```python
from build123d import *

# Parameters (mm, degrees)
ESBO_O1_W                        = 45
ESBO_O1_H                        = 45
RESSALTO_EXTRUS_O1_DEPTH         = 20
ESBO_O2_W                        = 25
ESBO_O2_H                        = 25
CORTE_EXTRUS_O1_DEPTH            = 70.705238631
ESBO_O3_W                        = 20
ESBO_O3_H                        = 20
RESSALTO_EXTRUS_O2_DEPTH         = 25
FURO_DE_DI_METRO_6_2_6_2_1_D     = 6.2
FURO_DE_DI_METRO_6_2_6_2_1_DEPTH = 35
FURO_DE_DI_METRO_6_2_6_2_2_D     = 6.2
FURO_DE_DI_METRO_6_2_6_2_2_DEPTH = 35
FURO_DE_DI_METRO_6_2_6_2_3_D     = 6.2
FURO_DE_DI_METRO_6_2_6_2_3_DEPTH = 35
FILETE2_R                        = 8
CHANFRO1_SIZE                    = 25
CHANFRO2_SIZE                    = 25
RESSALTO_EXTRUS_O3_DEPTH         = 20
ESBO_O12_R                       = 3
CORTE_EXTRUS_O2_DEPTH            = 71.906960985


# Some blends are built 0.0001 mm under size
with BuildPart() as part:
    # Esboço1 → Ressalto-extrusão1 (new body)
    with BuildSketch(Plane.XY.offset(20)):
        with Locations((-12.862035225, 34.142270059)):
            Rectangle(ESBO_O1_W, ESBO_O1_H)
    extrude(amount=-RESSALTO_EXTRUS_O1_DEPTH)

    # Esboço2 → Corte-extrusão1 (cut, through all)
    with BuildSketch(Plane(origin=(0, 0, 0), x_dir=(-1, 0, 0), z_dir=(0, 0, -1))):
        with Locations((2.862035225, 44.142270059)):
            Rectangle(ESBO_O2_W, ESBO_O2_H)
    extrude(amount=-CORTE_EXTRUS_O1_DEPTH, mode=Mode.SUBTRACT)

    # Esboço3 → Ressalto-extrusão2 (add)
    with BuildSketch(Plane.XY.offset(20)):
        with Locations((-25.362035225, 21.642270059)):
            Rectangle(ESBO_O3_W, ESBO_O3_H)
    extrude(amount=RESSALTO_EXTRUS_O2_DEPTH)

    # Furo de diâmetro Ø6.2 (6.2)1
    with Locations(Plane(origin=(9.637964775, 0, 0), x_dir=(0, 0, -1), z_dir=(1, 0, 0))):
        with Locations((-10, 21.642270059)):
            Hole(FURO_DE_DI_METRO_6_2_6_2_1_D / 2, depth=FURO_DE_DI_METRO_6_2_6_2_1_DEPTH)

    # Furo de diâmetro Ø6.2 (6.2)2
    with Locations(Plane(origin=(0, 56.642270059, 0), x_dir=(1, 0, 0), z_dir=(0, 1, 0))):
        with Locations((-25.362035225, -10)):
            Hole(FURO_DE_DI_METRO_6_2_6_2_2_D / 2, depth=FURO_DE_DI_METRO_6_2_6_2_2_DEPTH)

    # Furo de diâmetro Ø6.2 (6.2)3
    with Locations(Plane.XY.offset(45)):
        with Locations((-25.362035225, 21.642270059)):
            Hole(FURO_DE_DI_METRO_6_2_6_2_3_D / 2, depth=FURO_DE_DI_METRO_6_2_6_2_3_DEPTH)

    # Filete2
    filete2_edges = [part.edges().sort_by_distance(p)[0] for p in [
        (-35.362035225, 34.142270059, 0),
        (-12.862035225, 11.642270059, 0),
        (-35.362035225, 11.642270059, 22.5),
    ]]
    fillet(filete2_edges, radius=FILETE2_R)

    # Chanfro1
    # the kernel refuses this chamfer: 25 mm, written as the material it adds along each edge
    with BuildSketch(Plane(origin=(-35.362035225, 31.642270059, 20), x_dir=(0, -0.027495876610586317, 0.9996219169112966), z_dir=(1, 0, 0))) as chanfro1_piece_1_section:
        Polygon((CHANFRO1_SIZE * 0.999621916911, -CHANFRO1_SIZE * 0.0274958766106), (-CHANFRO1_SIZE * 0.0274958766106, -CHANFRO1_SIZE * 0.999621916911), (0, 0), align=None)
    chanfro1_piece_1 = extrude(amount=20, mode=Mode.PRIVATE)
    chanfro1_piece_1 = split(chanfro1_piece_1, bisect_by=Plane(origin=(-25.362035225, 39.873368248, 45), z_dir=(0, 0, -1)), keep=Keep.TOP, mode=Mode.PRIVATE)
    chanfro1_piece_1 = split(chanfro1_piece_1, bisect_by=Plane(origin=(-25.362035225, 56.642270059, 28.231098189), z_dir=(0, -1, 0)), keep=Keep.TOP, mode=Mode.PRIVATE)
    add(chanfro1_piece_1)

    # Chanfro2
    chanfro2_edges = [part.edges().sort_by_distance(p)[0] for p in [
        (-15.362035225, 31.642270059, 10),
    ]]
    chamfer(chanfro2_edges, length=CHANFRO2_SIZE - 0.0001)  # a hair under: the kernel refuses the full size

    # Esboço10 → Ressalto-extrusão3 (add)
    with BuildSketch(Plane.XZ.offset(-11.642270059)):
        Polygon((-15.362035225, 45), (9.637964775, 20), (-15.362035225, 20), align=None)
    extrude(amount=-RESSALTO_EXTRUS_O3_DEPTH)

    # Esboço12 → Corte-extrusão2 (cut, through all)
    with BuildSketch(Plane(origin=(20.426744945, 20.426744945, 20.426744945), x_dir=(-0.8164965809277259, 0.408248290463863, 0.4082482904638632), z_dir=(-0.577350269189626, -0.5773502691896256, -0.5773502691896258))):
        with Locations(Location((33.625917704, 8.232328107, 0), (0, 0, 120.000005232))):
            Circle(ESBO_O12_R)
    extrude(amount=CORTE_EXTRUS_O2_DEPTH, mode=Mode.SUBTRACT)


solid = part.part
```
Check sheet for the modelled part. Datum: model origin and axes. Units: mm. A direction names the side the tool comes from. Round coordinates to 2 decimals unless told otherwise and drop trailing zeros. Order: outer loops, then holes, each group sorted by start corner. A loop starts at its lowest first (then second) coordinate and runs counter-clockwise, first axis right, second up. Notation, with made-up numbers: M 12.5,34 L 52.5,34 A8 ccw 52.5,48 Z; hole C 58.25,-27.75 d9. An arc over 180 degrees is marked long. Answer in a Markdown table with one row per item.
(1) Section check B-B on y = 52.5. Record the boundary of the cut face in (x, z), plus the area to 3 significant figures.
Findings:
| item | result |
|---|---|
| outline | M -35.36,8 A8 ccw -27.36,0 L -11.22,0 L -11.22,20 L -15.36,20 L -15.36,24.14 L -35.36,24.14 Z; hole C -25.36,10 d6.2 |
| area | 522 mm^2 |
(2) Set-up check for faces 5 (the cylindrical face through (-28.226, 20.455, 27.58)), 6 (the cylindrical face through (-26.81, 15.99, 6.93)), 7 (the cylindrical face through (-7.782, 19.756, 7.54)), 8 (the flat face through (-8, 31.642, 27)), 9 (the cylindrical face through (-27.029, 39.222, 7.386)): record each of +Z, -Z, +X, -X, +Y, -Y from which the full face is reachable in a straight line by a thin tool's end or side.
Findings:
| item | result |
|---|---|
| face 5 | +Z |
| face 6 | none |
| face 7 | +X |
| face 8 | +Z, +X, +Y |
| face 9 | +Y |
(3) Gauge pin test, flat ends, axial feed: pin 1 (5 mm diameter, centred on y = 21.64, z = 10, fed in from +X); pin 2 (7 mm diameter, centred on x = -25.36, y = 21.64, fed in from +Z); pin 3 (12.5 mm diameter, centred on x = -6.5, z = 36, fed in from +Y); pin 4 (4 mm diameter, centred on x = -4, y = 46.5, fed in from +Z). Record the tip position at first contact, or that the pin passes through.
Findings:
| item | result |
|---|---|
| pin 1 | stops at x = -27.71 |
| pin 2 | stops at z = 45 |
| pin 3 | stops at y = 31.64 |
| pin 4 | stops at z = 20 |
(4) Material ranges on line 1 along Y through (x, z) = (-25.5, 16.5); line 2 along X through (y, z) = (37, 35); line 3 along Y through (x, z) = (-1.5, 10), recorded low to high. Write a range as from..to.
Findings:
| item | result |
|---|---|
| line 1 | y = 11.64..18.55, 24.74..56.64 |
| line 2 | x = -35.36..-15.36 |
| line 3 | y = 11.64..18.54, 24.74..42.78 |
(5) Draft check along X on faces 1 (the cylindrical face through (-16.33, 29.4, 14.89)), 2 (the cylindrical face through (-33.08, 14.05, 26.76)), 3 (the flat face through (-3.037, 21.502, 32.675)), 4 (the cylindrical face through (-8.6, 14.05, 2.28)). Enter one of: +X half, -X half, draft (parallel to the pull), parting line (faces both ways), or undercut.
Findings:
| item | result |
|---|---|
| face 1 | undercut |
| face 2 | -X half |
| face 3 | +X half |
| face 4 | draft |
